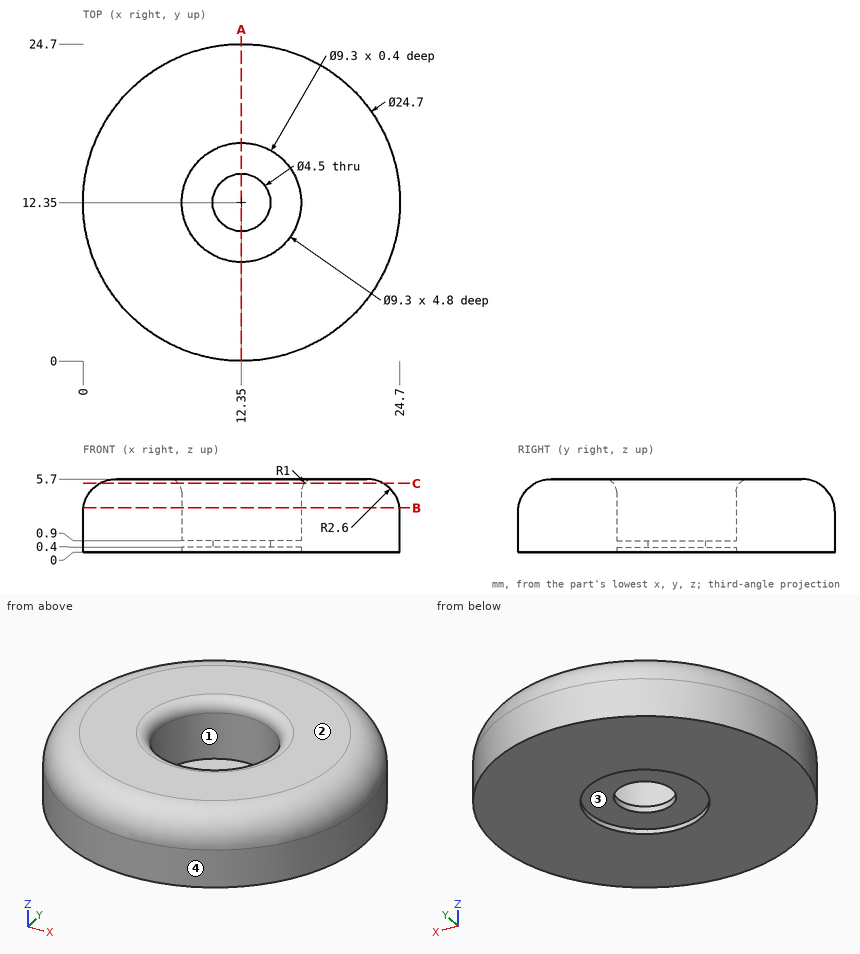
Could you check a few things on this drawing? It's one solid part, dimensions in mm from its lowest x, y, z. Coordinates: 2 decimals unless noted, no trailing zeros. Write each loop counter-clockwise with the first axis right and the second up, starting at its lowest first coordinate (ties: lowest second). Pieces come first, ordered by that corner, then holes.
Q1. If we mould it in two halves opening along Y, with no side actions, what happens to the marked faces 1, 2, 3 and 4? For each: +Y half, -Y half, draft (parallel to the pull), parting line (faces both ways), or undercut.
Results found:
face 1: undercut
face 2: draft
face 3: undercut
face 4: parting line
Q2. Imagine slicing it at C-C, the plane z = 5.35. List the corners of the cut face in (x, y) for me.
Results found:
outline: circle Ø22.11 at (12.35, 12.35); hole circle Ø9.78 at (12.35, 12.35)
Q3. Imagine slicing it at A-A, the plane x = 12.35. List the corners of the cut face in (y, z) for me, plus the area to 3 significant figures.
Results found:
outline: (0, 0) - (7.7, 0) - (7.7, 0.4) - (10.1, 0.4) - (10.1, 0.9) - (7.7, 0.9) - (7.7, 4.7) arc R1 ccw to (6.7, 5.7) - (2.6, 5.7) arc R2.6 ccw to (0, 3.1) - close; (14.6, 0.4) - (17, 0.4) - (17, 0) - (24.7, 0) - (24.7, 3.1) arc R2.6 ccw to (22.1, 5.7) - (18, 5.7) arc R1 ccw to (17, 4.7) - (17, 0.9) - (14.6, 0.9) - close
area: 86.8 mm2
Q4. Imagine slicing it at B-B, the plane z = 3.45. List the corners of the cut face in (x, y) for me, plus the area to 3 significant figures.
Results found:
outline: circle Ø24.65 at (12.35, 12.35); hole circle Ø9.3 at (12.35, 12.35)
area: 409 mm2
Q5. For P1, Ø1, axis at y = 6, z = 2, coming from the -X side; P2, Ø2, axis at y = 16.5, z = 2.5, coming from the -X side; P3, Ø2, axis at x = 15.5, z = 1.5, coming from the +Y side; P4, Ø3.5, axis at x = 12.35, y = 12.35, coming from the -Z side, each with a flat end and sliding along its axis, tell me the tip position at first contact or that it passes through.
Results found:
P1: stops at x = 1.47
P2: stops at x = 0.41
P3: stops at y = 24.51
P4: passes through
Q6. Please list where these lines run through material, in increasing order: L1, parallel to Y at x = 12.35, z = 0.3; L2, parallel to Y at x = 16, z = 1.8; L3, parallel to X at y = 10.25, z = 3.6.
Results found:
L1: y = 0 to 7.7, 17 to 24.7
L2: y = 0.55 to 9.47, 15.23 to 24.15
L3: x = 0.23 to 8.2, 16.5 to 24.47
